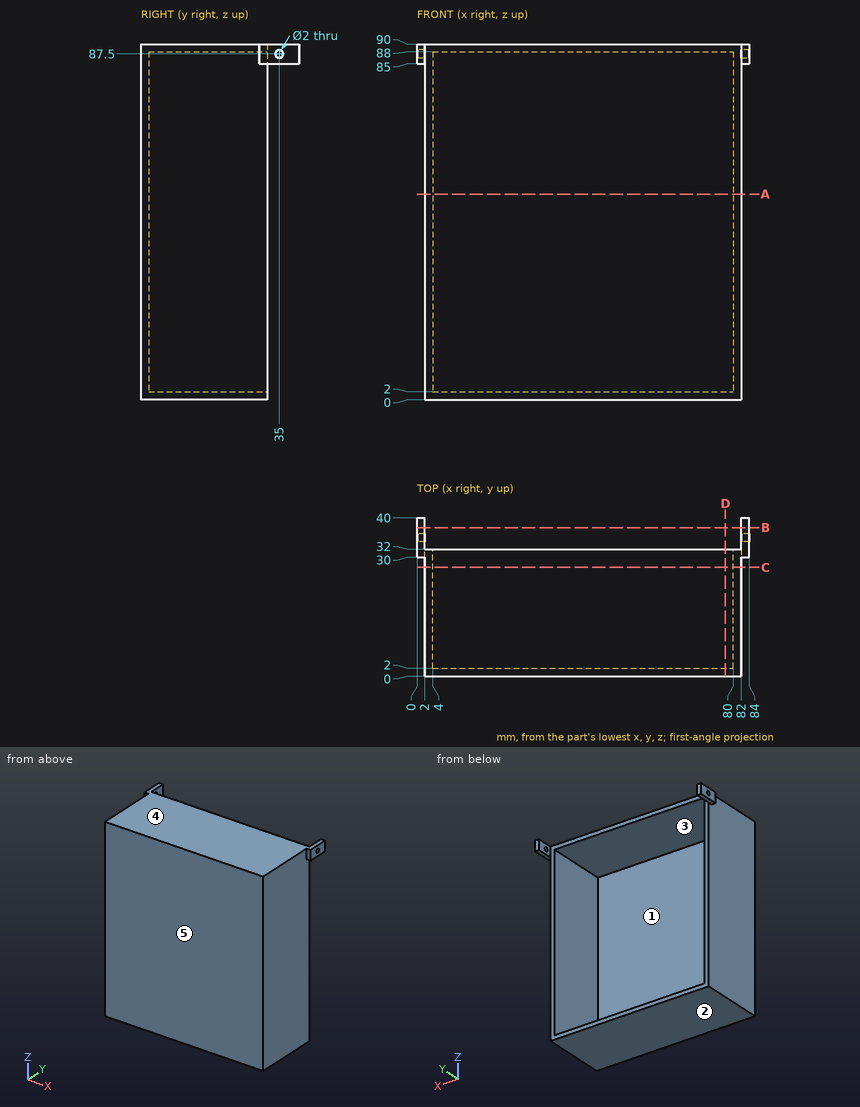
The drawing under review shows one solid part. Ordinate dimensions are in mm from its lowest x, y, z. A direction names the side the tool comes from. Round coordinates to 2 decimals unless told otherwise and drop trailing zeros. Write each loop counter-clockwise with the first axis right and the second up, starting at its lowest first coordinate (ties: lowest second). Pieces come first, ordered by that corner, then holes.
(1) Insertion check: pin 1 (9 mm diameter, centred on y = 18.5, z = 65, fed in from -X); pin 2 (1 mm diameter, centred on y = 5.5, z = 20, fed in from +X); pin 3 (2 mm diameter, centred on x = 0.5, z = 88, fed in from -Y). Each pin has a flat end and moves straight along its axis. Give the tip position at first contact, or say it passes through.
(2) We need section B-B on y = 37.5. Give the boundary of the cut face in (x, z), and give its area (3 significant figures).
(3) Wall thickness on L1, parallel to Z at x = 9, y = 18; L2, parallel to X at y = 31, z = 14; L3, parallel to Z at x = 0.4, y = 35: over which ranges is each line inside the solid? List them lowest first.
(4) Mouldability with a two-part tool opening along Z and no side actions: class the marked faces 3, 4 and 5 as +Z half, -Z half, draft (parallel to the pull), parting line (faces both ways), or undercut.
(5) Machinability: for the marked faces 1 and 2, which of the approach directions +Z, -Z, +X, -X, +Y, -Y give a long, thin tool a straight path to every point of the face, cutting with its end or side? Answer none if there is none.
(6) We need section A-A on z = 52. Give the boundary of the cut face in (x, y).
(7) We need section C-C on y = 27.5. Give the boundary of the cut face in (x, z).
(8) We need section D-D on x = 78. Give the boundary of the cut face in (y, z).
Findings below:
1. pin 1: stops at x = 2
1. pin 2: stops at x = 82
1. pin 3: stops at y = 30
2. outline: (0, 85) - (2, 85) - (2, 90) - (0, 90) - close; (82, 85) - (84, 85) - (84, 90) - (82, 90) - close
2. area: 20.0 mm2
3. L1: z = 0 to 2, 88 to 90
3. L2: x = 2 to 4, 80 to 82
3. L3: z = 85 to 86.5, 88.5 to 90
4. face 3: undercut
4. face 4: +Z half
4. face 5: draft
5. face 1: +Y
5. face 2: -Z, +X, -X, +Y, -Y
6. outline: (2, 0) - (82, 0) - (82, 32) - (80, 32) - (80, 2) - (4, 2) - (4, 32) - (2, 32) - close
7. outline: (2, 0) - (82, 0) - (82, 90) - (2, 90) - close; hole (4, 2) - (80, 2) - (80, 88) - (4, 88) - close
8. outline: (0, 0) - (32, 0) - (32, 2) - (2, 2) - (2, 88) - (32, 88) - (32, 90) - (0, 90) - close
